For this review, take the finished solid that the model builds, in its own axes (mm). A direction names the side the tool comes from. Coordinates: 2 decimals unless noted, no trailing zeros. Write each loop counter-clockwise with the first axis right and the second up, starting at its lowest first coordinate (ties: lowest second). Pieces come first, ordered by that corner, then holes. Notation, with made-up numbers: M 81,36 L 128,36 A25 ccw 128,53 Z; hole C 81,-9 d10. An arc over 180 degrees is marked long. One line per question, with ' | ' between items.
from build123d import *

# Parameters (mm, degrees)
F1_DEPTH = 76.2
F2_R     = 5.08


with BuildPart() as f1:
    # F0 (on Front) → F1 (new body)
    with BuildSketch(Plane.XZ):
        Polygon((0, 28.445911), (0, -60.454089), (19.05, -60.454089), (19.05, 66.545911), (0, 66.545911), (0, 47.495911), (9.525, 47.495911), (9.525, 28.445911), align=None)
    extrude(amount=F1_DEPTH)

    # F2
    f2_edges = [f1.edges().sort_by_distance(p)[0] for p in [
        (0, -76.2, -16.004089),
        (0, 0, -16.004089),
        (9.525, -76.2, 66.545911),
        (0, -38.1, 66.545911),
        (19.05, -76.2, 3.045911),
        (19.05, -38.1, 66.545911),
        (9.525, 0, 66.545911),
        (19.05, 0, 3.045911),
        (0, 0, 57.020911),
        (0, -76.2, 57.020911),
    ]]
    fillet(f2_edges, radius=F2_R)


solid = f1.part
1) We need section A-A on x = 8.25. State the section outline as (y, z) points.
Responses:
outline: M -76.2,-60.45 L 0,-60.45 L 0,28.45 L -76.2,28.45 Z; M -76.2,47.5 L 0,47.5 L 0,61.47 A5.08 ccw -5.08,66.55 L -71.12,66.55 A5.08 ccw -76.2,61.47 Z
2) Machinability: for faces 4 (the flat face through (0, -38, 55)), 5 (the flat face through (9.525, -38, 38)), which of the approach directions +Z, -Z, +X, -X, +Y, -Y give a long, thin tool a straight path to every point of the face, cutting with its end or side? Answer none if there is none.
Responses:
face 4: +Z, -Z, -X, +Y, -Y | face 5: -X, +Y, -Y
3) We need section C-C on y = -22. State the section outline as (x, z) points (3 decimals).
Responses:
outline: M 0,-60.454 L 19.05,-60.454 L 19.05,61.466 A5.08 ccw 13.97,66.546 L 5.08,66.546 A5.08 ccw 0,61.466 L 0,47.496 L 9.525,47.496 L 9.525,28.446 L 0,28.446 Z
4) We need section D-D on x = 2. State the section outline as (y, z) points, then the cut area to 3 significant figures.
Responses:
outline: M -75.16,-60.45 L -1.04,-60.45 L -1.04,28.45 L -75.16,28.45 Z; M -75.16,47.5 L -1.04,47.5 L -1.04,61.47 A4.04 ccw -5.08,65.51 L -71.12,65.51 A4.04 ccw -75.16,61.47 Z | area: 7,920 mm^2
5) We need section B-B on z = 12.5. State the section outline as (x, y) points, then the cut area to 3 significant figures.
Responses:
outline: M 0,-71.12 A5.08 ccw 5.08,-76.2 L 13.97,-76.2 A5.08 ccw 19.05,-71.12 L 19.05,-5.08 A5.08 ccw 13.97,0 L 5.08,0 A5.08 ccw 0,-5.08 Z | area: 1,430 mm^2
6) The part is to be moulded in two halves that separate along Z. For faces 1 (the flat face through (0, -38, -15)), 2 (the flat face through (5, -38, 28.446)), 3 (the cylindrical face through (9.46, -74.67, 65.1)), say which applies: +Z half, -Z half, draft (parallel to the pull), parting line (faces both ways), or undercut.
Responses:
face 1: draft | face 2: undercut | face 3: +Z half
7) To check wall thickness, follow line 1 along Z through (x, y) = (5, -13); line 2 along X through (y, z) = (-57.5, 40) (3 decimals). State the ranges of each line that lie inside material, in increasing order. Write a range as [from, to].
Responses:
line 1: [-60.45, 28.45], [47.5, 66.55] | line 2: [9.525, 19.05]
8) Insertion check: pin 1 Ø5.5 at (y, z) = (-27, 34) entering from -X (3 decimals); pin 2 Ø2 at (x, z) = (3, 6.5) entering from +Y. Each pin has a flat end and moves straight along its axis. Give the tip position at first contact, or say it passes through.
Responses:
pin 1: x = 9.525 | pin 2: y = -0.12
